```python
from build123d import *

# Parameters (mm, degrees)
BOSS_EXTRUDE1_DEPTH = 20
SKETCH2_R           = 3.5
CUT_EXTRUDE1_DEPTH  = 4
FILLET1_R           = 2


with BuildPart() as part:
    # Sketch1 → Boss-Extrude1 (new body)
    with BuildSketch(Plane(origin=(0, 0, 0), x_dir=(0, 0, -1), z_dir=(1, 0, 0))):
        Polygon((-10.5, 0), (10.5, 0), (10.5, -14), (33.5, -14), (33.5, -10), (14.5, -10), (14.5, 4), (-14.5, 4), (-14.5, -10), (-33.5, -10), (-33.5, -14), (-10.5, -14), align=None)
    extrude(amount=BOSS_EXTRUDE1_DEPTH)

    # Sketch2 → Cut-Extrude1 (cut)
    with BuildSketch(Plane(origin=(0, -10, 0), x_dir=(1, 0, 0), z_dir=(0, 1, 0))):
        with Locations(Location((10, 24, 0), (0, 0, 270))):
            Circle(SKETCH2_R)
    cut_extrude1 = extrude(amount=-CUT_EXTRUDE1_DEPTH, mode=Mode.SUBTRACT)

    # Mirror1: Cut-Extrude1 across plane
    add(cut_extrude1.mirror(Plane.XY), mode=Mode.SUBTRACT)

    # Fillet1
    fillet1_edges = [part.edges().sort_by_distance(p)[0] for p in [
        (0, 4, 0),
        (10, -14, 10.5),
        (10, -10, 14.5),
        (10, 4, 14.5),
        (10, 4, -14.5),
        (10, -10, -14.5),
        (10, -14, -10.5),
        (10, 0, -10.5),
        (10, 0, 10.5),
        (20, 4, 0),
    ]]
    fillet(fillet1_edges, radius=FILLET1_R)


solid = part.part
```
The model under review builds one solid part; all positions refer to its coordinate system, in mm. A direction names the side the tool comes from. Round coordinates to 2 decimals unless told otherwise and drop trailing zeros. Order: outer loops, then holes, each group sorted by start corner. A loop starts at its lowest first (then second) coordinate and runs counter-clockwise, first axis right, second up.
(1) Take a section at C-C, the plane x = 10. State the section outline as (y, z) points.
Working result:
outline: (-14, -33.5) - (-10, -33.5) - (-10, -27.5) - (-14, -27.5) - close; (-14, -20.5) - (-10, -20.5) - (-10, -16.5) arc R2 cw to (-8, -14.5) - (2, -14.5) arc R2 ccw to (4, -12.5) - (4, 12.5) arc R2 ccw to (2, 14.5) - (-8, 14.5) arc R2 cw to (-10, 16.5) - (-10, 20.5) - (-14, 20.5) - (-14, 12.5) arc R2 ccw to (-12, 10.5) - (-2, 10.5) arc R2 cw to (0, 8.5) - (0, -8.5) arc R2 cw to (-2, -10.5) - (-12, -10.5) arc R2 ccw to (-14, -12.5) - close; (-14, 27.5) - (-10, 27.5) - (-10, 33.5) - (-14, 33.5) - close
(2) Tool access review of faces 1 (the face through (10, -3, -14.5)), 2 (the face through (7.6, -10, 26.8)), 3 (the face through (10, -7, 10.5)), 4 (the face through (19.43, 3.4, 0.2)): name each direction out of +Z, -Z, +X, -X, +Y, -Y from which nothing blocks a thin tool from reaching the whole face with its end or side.
Working result:
face 1: -Z, +X, -X, +Y
face 2: +Z, +X, -X, +Y
face 3: +X, -X, -Y
face 4: +Z, -Z, +X, +Y
(3) Mouldability with a two-part tool opening along Z and no side actions: class faces 5 (the face through (20, 1, 3)), 6 (the face through (10.14, 3.43, 13.9)), 7 (the face through (6.895, -11.972, 22.385)) as released by +Z, released by -Z, zero draft, split by the parting line, or undercut.
Working result:
face 5: zero draft
face 6: released by +Z
face 7: undercut
(4) For P1, Ø9, axis at x = 10, z = 24, coming from the +Y side; P2, Ø6, axis at x = 13.5, y = -3.5, coming from the +Z side; P3, Ø3, axis at x = 10.5, y = -3.5, coming from the -Z side; P4, Ø10, axis at y = -8.5, z = 4, coming from the -X side, all flat-tipped, find the tip position at first contact; note any pin that passes through.
Working result:
P1: stops at y = -10
P2: stops at z = 14.5
P3: stops at z = -14.5
P4: passes through
(5) Take a section at A-A, the plane z = -24. State the section outline as (x, y) points.
Working result:
outline: (0, -14) - (6.5, -14) - (6.5, -10) - (0, -10) - close; (13.5, -14) - (20, -14) - (20, -10) - (13.5, -10) - close
(6) Take a section at D-D, the plane x = 16.5. State the section outline as (y, z) points.
Working result:
outline: (-14, -33.5) - (-10, -33.5) - (-10, -16.5) arc R2 cw to (-8, -14.5) - (2, -14.5) arc R2 ccw to (4, -12.5) - (4, 12.5) arc R2 ccw to (2, 14.5) - (-8, 14.5) arc R2 cw to (-10, 16.5) - (-10, 33.5) - (-14, 33.5) - (-14, 12.5) arc R2 ccw to (-12, 10.5) - (-2, 10.5) arc R2 cw to (0, 8.5) - (0, -8.5) arc R2 cw to (-2, -10.5) - (-12, -10.5) arc R2 ccw to (-14, -12.5) - close
(7) Wall thickness on L1, parallel to X at y = -12, z = -24; L2, parallel to Z at x = 19, y = -11.5; L3, parallel to Z at x = 2, y = -4: over which ranges is each line inside the solid? List them lowest first.
Working result:
L1: x = 0 to 6.5, 13.5 to 20
L2: z = -33.5 to -10.5, 10.5 to 33.5
L3: z = -14.5 to -10.5, 10.5 to 14.5
(8) Take a section at B-B, the plane y = -3.5. State the section outline as (x, z) points.
Working result:
outline: (0, -14.5) - (20, -14.5) - (20, -10.5) - (0, -10.5) - close; (0, 10.5) - (20, 10.5) - (20, 14.5) - (0, 14.5) - close
